The model under review builds one solid part; all positions refer to its coordinate system, in mm. Face numbers are marked on the shaded views. A direction names the side the tool comes from. Coordinates: 2 decimals unless noted, no trailing zeros. Write each loop counter-clockwise with the first axis right and the second up, starting at its lowest first coordinate (ties: lowest second). Pieces come first, ordered by that corner, then holes. Notation, with made-up numbers: (59.5, 23) - (79.5, 23) arc R11 cw to (79.5, 28) - close; hole circle Ø9 at (-27, 84). An arc over 180 degrees is marked (long way). Return JSON: item names as keys, results as strings. Group by question number.
(1) Draft analysis for pull direction Z (two halves, no side actions). For the marked faces 1, 2 and 3, state which applies: released by +Z, released by -Z, zero draft, split by the parting line, or undercut.
(2) We need section B-B on z = 5.5. State the section outline as (x, y) points, then the cut area to 3 significant figures.
(3) We need section A-A on x = 40. State the section outline as (y, z) points.
(4) To check wall thickness, follow L1, parallel to Z at x = 40, y = -11.25; L2, parallel to X at y = -13.75, z = -6; L3, parallel to X at y = -15.5, z = 11.75. State the ranges of each line that lie inside material, in increasing order. Write a range as from..to.
(5) We need section D-D on y = -2.25. State the section outline as (x, z) points.
(6) Tool access review of the marked faces 4, 5 and 6: name each direction out of +Z, -Z, +X, -X, +Y, -Y from which nothing blocks a thin tool from reaching the whole face with its end or side.
(7) For pin 1 Ø9 at (x, z) = (6.5, -1.5) entering from -Y; pin 2 Ø8 at (x, y) = (-17, -11) entering from +Z; pin 3 Ø8 at (x, z) = (-47, 0.5) entering from -Y; pin 4 Ø12 at (x, z) = (40, -0.89) entering from -Y, all flat-tipped, find the tip position at first contact; note any pin that passes through.
(8) We need section C-C on z = 12.25. State the section outline as (x, y) points, then the cut area to 3 significant figures.
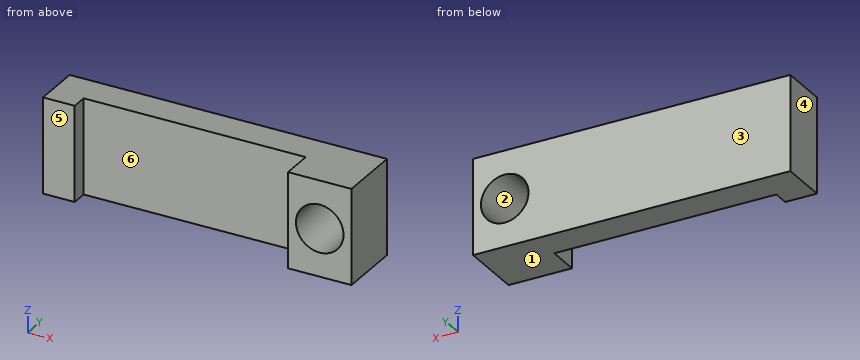
```python
from build123d import *

# Parameters (mm, degrees)
F0_W     = 100
F0_H     = 30
F1_DEPTH = 10
F2_W     = 10
F2_H     = 30
F3_DEPTH = 5
F4_W     = 20
F4_H     = 30
F5_DEPTH = 10
F6_R     = 7.5
F7_DEPTH = 20.001


with BuildPart() as f1:
    # F0 (on Front) → F1 (new body)
    with BuildSketch(Plane.XZ):
        with Locations((0, -0.888889)):
            Rectangle(F0_W, F0_H)
    extrude(amount=F1_DEPTH)

    # F2 (on face) → F3 (join)
    with BuildSketch(Plane.XZ.offset(10)):
        with Locations((-45, -0.888889)):
            Rectangle(F2_W, F2_H)
    extrude(amount=F3_DEPTH)

    # F4 (on face) → F5 (join)
    with BuildSketch(Plane.XZ.offset(10)):
        with Locations((40, -0.888889)):
            Rectangle(F4_W, F4_H)
    extrude(amount=F5_DEPTH)

    # F6 (on face) → F7 (cut, through all)
    with BuildSketch(Plane.XZ.offset(20)):
        with Locations((40, -0.888889)):
            Circle(F6_R)
    extrude(amount=-F7_DEPTH, mode=Mode.SUBTRACT)


solid = f1.part
```
Ans:
{
 "1": {"face 1": "released by -Z", "face 2": "undercut", "face 3": "zero draft"},
 "2": {"outline": "(-50, -15) - (-40, -15) - (-40, -10) - (30, -10) - (30, -20) - (36.07, -20) - (36.07, 0) - (-50, 0) - close; (43.93, -20) - (50, -20) - (50, 0) - (43.93, 0) - close", "area": "1,090 mm²"},
 "3": {"outline": "(-20, -15.89) - (0, -15.89) - (0, -8.39) - (-20, -8.39) - close; (-20, 6.61) - (0, 6.61) - (0, 14.11) - (-20, 14.11) - close"},
 "4": {"L1": "-15.89..-8.39, 6.61..14.11", "L2": "-50..-40, 30..34.51, 45.49..50", "L3": "30..50"},
 "5": {"outline": "(-50, -15.89) - (50, -15.89) - (50, 14.11) - (-50, 14.11) - close; hole circle Ø15 at (40, -0.89)"},
 "6": {"face 4": "+Z, -Z, -X, +Y, -Y", "face 5": "+Z, -Z, -X, -Y", "face 6": "+Z, -Z, -Y"},
 "7": {"pin 1": "y = -10", "pin 2": "z = 14.11", "pin 3": "y = -15", "pin 4": "through"},
 "8": {"outline": "(-50, -15) - (-40, -15) - (-40, -10) - (30, -10) - (30, -20) - (50, -20) - (50, 0) - (-50, 0) - close", "area": "1,250 mm²"}
}
